Can you work these out from the model? Positions are in its coordinate system, mm. Face numbers are marked on the shaded views. A direction names the side the tool comes from. Give positions to 0.01 mm unless a question says otherwise; leave off trailing zeros. Order: outer loops, then holes, each group sorted by start corner. A loop starts at its lowest first (then second) coordinate and runs counter-clockwise, first axis right, second up.
Item 1: I'm going to push flat-ended pins straight in: pin 1 Ø3 at (x, y) = (1, 7) entering from -Z; pin 2 Ø2.5 at (x, z) = (-4.5, -30) entering from +Y; pin 3 Ø1 at (y, z) = (7.5, 26) entering from -X. Where does each tip first touch, or does it pass through?
Item 2: I want a section at C-C, the plane y = 4. Write out the boundary of the cut face in (x, z), then the cut area to 3 significant figures.
Item 3: I want a section at D-D, the plane z = 30. Write out the boundary of the cut face in (x, y).
Item 4: Which directions (+Z, -Z, +X, -X, +Y, -Y) give clear straight access to the entire face, cutting with the end or side of a thin tool? Please do the marked faces 1 and 2.
Item 5: I want a section at B-B, the plane z = -30.5. Write out the boundary of the cut face in (x, y), then the cut area to 3 significant figures.
Item 6: I want a section at A-A, the plane x = 0. Write out the boundary of the cut face in (y, z).
Item 7: If I drill on line 1 along X through (y, z) = (1.25, -30.5); line 2 along Z through (x, y) = (9, 3.5); line 3 along Z through (x, y) = (5, 1.25), over which ranges is the centre line in solid material (lowest first)?
```python
from build123d import *

# Parameters (mm, degrees)
SKETCH1_R           = 1.75
BOSS_EXTRUDE1_DEPTH = 11
SKETCH2_W           = 27.712142642
SKETCH2_H           = 8.5
CUT_EXTRUDE1_DEPTH  = 8


with BuildPart() as part:
    # Sketch1 → Boss-Extrude1 (new body)
    with BuildSketch(Plane(origin=(0, 0, 0), x_dir=(1, 0, 0), z_dir=(0, 1, 0))):
        with BuildLine():
            Line((17, -27.5), (10.712142643, -27.5))
            ThreePointArc((10.712142643, -27.5), (7.29344406, -28.691578015), (5.356071321, -31.75))
            ThreePointArc((5.356071321, -31.75), (0, -36), (-5.356071321, -31.75))
            ThreePointArc((-5.356071321, -31.75), (-7.29344406, -28.691578015), (-10.712142643, -27.5))
            Line((-10.712142643, -27.5), (-17, -27.5))
            ThreePointArc((-17, -27.5), (-20.535533906, -26.035533906), (-22, -22.5))
            Line((-22, -22.5), (-22, 22.5))
            ThreePointArc((-22, 22.5), (-20.535533906, 26.035533906), (-17, 27.5))
            Line((-17, 27.5), (-10.712142643, 27.5))
            ThreePointArc((-10.712142643, 27.5), (-7.29344406, 28.691578015), (-5.356071321, 31.75))
            ThreePointArc((-5.356071321, 31.75), (0, 36), (5.356071321, 31.75))
            ThreePointArc((5.356071321, 31.75), (7.29344406, 28.691578015), (10.712142643, 27.5))
            Line((10.712142643, 27.5), (17, 27.5))
            ThreePointArc((17, 27.5), (20.535533906, 26.035533906), (22, 22.5))
            Line((22, 22.5), (22, -22.5))
            ThreePointArc((22, -22.5), (20.535533906, -26.035533906), (17, -27.5))
        make_face()
        with Locations(Location((0, -30.5, 0), (0, 0, 270))):
            Circle(SKETCH1_R, mode=Mode.SUBTRACT)
        with Locations(Location((0, 30.5, 0), (0, 0, 270))):
            Circle(SKETCH1_R, mode=Mode.SUBTRACT)
    extrude(amount=BOSS_EXTRUDE1_DEPTH)

    # Sketch2 → Cut-Extrude1 (cut)
    with BuildSketch(Plane(origin=(0, 11, 0), x_dir=(1, 0, 0), z_dir=(0, 1, 0))):
        with Locations((0, -31.75)):
            Rectangle(SKETCH2_W, SKETCH2_H)
        with Locations((0, 31.75)):
            Rectangle(SKETCH2_W, SKETCH2_H)
    extrude(amount=-CUT_EXTRUDE1_DEPTH, mode=Mode.SUBTRACT)


solid = part.part
```
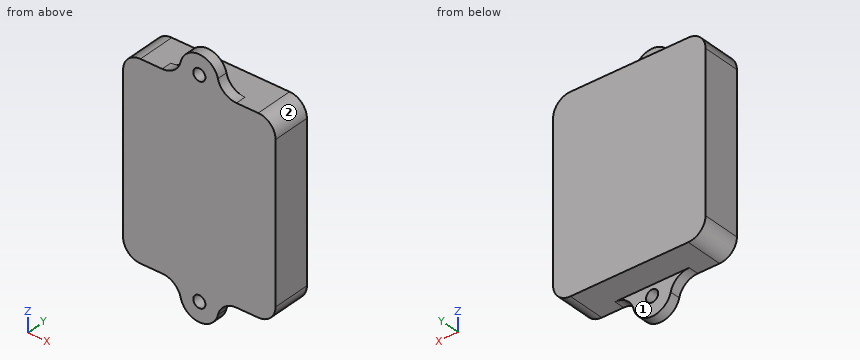
Results list:
1. pin 1: stops at z = -27.5
1. pin 2: stops at y = 3
1. pin 3: stops at x = -21
2. outline: (-22, -22.5) arc R5 ccw to (-17, -27.5) - (17, -27.5) arc R5 ccw to (22, -22.5) - (22, 22.5) arc R5 ccw to (17, 27.5) - (-17, 27.5) arc R5 ccw to (-22, 22.5) - close
2. area: 2,400 mm2
3. outline: (-6.1, 0) - (-1.68, 0) - (-1.68, 3) - (-6.1, 3) - close; (1.68, 0) - (6.1, 0) - (6.1, 3) - (1.68, 3) - close
4. face 1: -Z, +X, -X, +Y
4. face 2: +Z, +X, +Y, -Y
5. outline: (-5.81, 0) - (-1.75, 0) - (-1.75, 3) - (-5.81, 3) - close; (1.75, 0) - (5.81, 0) - (5.81, 3) - (1.75, 3) - close
5. area: 24.4 mm2
6. outline: (0, -36) - (3, -36) - (3, -32.25) - (0, -32.25) - close; (0, -28.75) - (3, -28.75) - (3, -27.5) - (11, -27.5) - (11, 27.5) - (3, 27.5) - (3, 28.75) - (0, 28.75) - close; (0, 32.25) - (3, 32.25) - (3, 36) - (0, 36) - close
7. line 1: x = -5.81 to -1.75, 1.75 to 5.81
7. line 2: z = -27.5 to 27.5
7. line 3: z = -32.79 to 32.79
